from build123d import *

# Parameters (mm, degrees)
BOSS_EXTRUDE1_DEPTH = 3
BOSS_EXTRUDE2_START = -3
BOSS_EXTRUDE2_DEPTH = 3
SKETCH3_R           = 1.6
CUT_EXTRUDE1_DEPTH  = 49.760896398
BOSS_EXTRUDE3_START = 10
BOSS_EXTRUDE3_DEPTH = 10
BOSS_EXTRUDE4_DEPTH = 15


with BuildPart() as part:
    # Sketch1 → Boss-Extrude1 (new body)
    with BuildSketch(Plane(origin=(0, 0, 0), x_dir=(1, 0, 0), z_dir=(0, 1, 0))):
        with BuildLine():
            Line((2.5, 0), (2.5, -16.552945357))
            ThreePointArc((2.5, -16.552945357), (0, -19.052945357), (-2.5, -16.552945357))
            Line((-2.5, -16.552945357), (-2.5, 0))
            ThreePointArc((-2.5, 0), (0, 2.5), (2.5, 0))
        make_face()
    extrude(amount=BOSS_EXTRUDE1_DEPTH)

    # Sketch2 → Boss-Extrude2 (add)
    with BuildSketch(Plane(origin=(0, 3, 0), x_dir=(1, 0, 0), z_dir=(0, 1, 0)).offset(BOSS_EXTRUDE2_START)):
        with BuildLine():
            Line((2.26545785, -15.495731694), (14.95202181, -42.681225894))
            ThreePointArc((14.95202181, -42.681225894), (13.743777623, -46.003897407), (10.42110611, -44.79565322))
            Line((10.42110611, -44.79565322), (-2.26545785, -17.610159021))
            ThreePointArc((-2.26545785, -17.610159021), (-1.057213663, -14.287487507), (2.26545785, -15.495731694))
        make_face()
    extrude(amount=BOSS_EXTRUDE2_DEPTH)

    # Sketch3 → Cut-Extrude1 (cut, through all)
    with BuildSketch(Plane(origin=(0, 3, 0), x_dir=(1, 0, 0), z_dir=(0, 1, 0))):
        with Locations(Location((0, 0, 0), (0, 0, 270))):
            Circle(SKETCH3_R)
        with Locations(Location((0, -16.552945357, 0), (0, 0, 270))):
            Circle(SKETCH3_R)
    extrude(amount=-CUT_EXTRUDE1_DEPTH, mode=Mode.SUBTRACT)

    # Sketch5 → Boss-Extrude3 (add)
    with BuildSketch(Plane.XZ.offset(BOSS_EXTRUDE3_START)):
        with BuildLine():
            Line((14.95202181, 42.681225894), (6.494312503, 24.557563094))
            ThreePointArc((6.494312503, 24.557563094), (3.171640989, 23.349318908), (1.963396803, 26.671990421))
            Line((1.963396803, 26.671990421), (10.42110611, 44.795653221))
            ThreePointArc((10.42110611, 44.795653221), (13.743777623, 46.003897407), (14.95202181, 42.681225894))
        make_face()
    extrude(amount=-BOSS_EXTRUDE3_DEPTH)

    # Sketch6 → Boss-Extrude4 (add)
    with BuildSketch(Plane(origin=(0, 3, 0), x_dir=(1, 0, 0), z_dir=(0, 1, 0))):
        with BuildLine():
            Line((10.42110611, -44.79565322), (1.963396803, -26.671990421))
            ThreePointArc((1.963396803, -26.671990421), (3.17164099, -23.349318907), (6.494312503, -24.557563094))
            Line((6.494312503, -24.557563094), (14.95202181, -42.681225894))
            ThreePointArc((14.95202181, -42.681225894), (13.743777623, -46.003897407), (10.42110611, -44.79565322))
        make_face()
    extrude(amount=BOSS_EXTRUDE4_DEPTH)


solid = part.part
Geometry: final body of the model. Coordinates: model frame, mm. A direction names the side the tool comes from. Coordinates: 2 decimals unless noted, no trailing zeros. Loops run counter-clockwise (first coordinate to the right, second up) from the corner with the lowest first, then second, coordinate; pieces in that order, holes last. Notation, with made-up numbers: (-15, -19.5) - (20, -19.5) arc R21 cw to (20, -5.5) - close; hole circle Ø2 at (80.5, 47). An arc over 180 degrees is marked (long way). Put each result on its own line as item: value. Start each with the question number.
Q1. Set-up query: faces 1 (the flat face through (2.5, 1, 8)), 2 (the cylindrical face through (-2.44, 1.48, 17.1)). Return all of +Z, -Z, +X, -X, +Y, -Y with unobstructed straight access to the full face (end or side cutting, diameter ignored); none if empty.
Q2. Pin query (flat end, axial travel): pin 1 Ø6 at (x, y) = (12.5, 1) entering from -Z; pin 2 Ø1 at (x, y) = (4, 5.5) entering from -Z; pin 3 Ø3 at (x, z) = (0.5, 9) entering from +Y. Return the tip coordinate at first contact, or that it passes through.
Q3. Cut plane B-B, the plane x = 5. Return loops of the section in (y, z), and give its area (3 significant figures).
Q4. Pull-direction query (Z, two-part tool) for faces 3 (the cylindrical face through (3.222, -5.07, 23.327)), 4 (the cylindrical face through (-0.1, 1.5, -2.5)), 5 (the cylindrical face through (-0.97, 1.52, -1.27)); classes: released by +Z, released by -Z, zero draft, split by the parting line, or undercut.
Q5. Cut plane A-A, the plane x = -0.5. Return loops of the section in (y, z), and give its area (3 significant figures).
Q6. Cut plane C-C, the plane z = 42. Return loops of the section in (x, y).
Q7. Cut plane D-D, the plane y = 5.5. Return loops of the section in (x, z).
Q8. Line query: line 1 (Y direction, x = 2, z = 23); line 2 (X direction, y = 0.5, z = 20); line 3 (X direction, y = 0.75, z = 5). Output: solid intervals per line, ascending.
Filled sheet:
1. face 1: -Z, +X, +Y, -Y
1. face 2: +Z, -X, +Y, -Y
2. pin 1: z = 31
2. pin 2: z = 23.11
2. pin 3: y = 3
3. outline: (-10, 23.24) - (0, 23.24) - (0, 21.36) - (3, 21.36) - (3, 23.24) - (18, 23.24) - (18, 33.18) - (-10, 33.18) - close
3. area: 284 mm²
4. face 3: split by the parting line
4. face 4: released by -Z
4. face 5: undercut
5. outline: (0, -2.45) - (3, -2.45) - (3, -1.52) - (0, -1.52) - close; (0, 1.52) - (3, 1.52) - (3, 15.03) - (0, 15.03) - close; (0, 18.07) - (3, 18.07) - (3, 21.39) - (0, 21.39) - close
5. area: 53.3 mm²
6. outline: (9.12, -10) - (14.63, -10) - (14.63, 18) - (9.12, 18) - close
7. outline: (1.96, 26.67) arc R2.5 ccw to (6.49, 24.56) - (14.95, 42.68) arc R2.5 ccw to (10.42, 44.8) - close
8. line 1: 0 to 3
8. line 2: -1.15 to 4.37
8. line 3: -2.5 to 2.5
